Geometry check sheet. Reference: the model listing, model coordinates, mm. A direction names the side the tool comes from. Coordinates: 2 decimals unless noted, no trailing zeros. Write each loop counter-clockwise with the first axis right and the second up, starting at its lowest first coordinate (ties: lowest second). Pieces come first, ordered by that corner, then holes.
Autodesk Fusion 360 part; units mm, degrees
sketch "Sketch1" plane through (0, 0, 0) normal (0, 0, 1) x (1, 0, 0)
  circle A0 centre (0, 0) radius 23
  circle A1 centre (0, 0) radius 14
  circle A2 centre (0, 0) radius 17
  dimension "d1" = 46
  dimension "d2" = 28
  dimension "d3" = 34
extrude "Extrude1" add sketch "Sketch1" along normal blind 3 contours A0 | A2
extrude "Extrude2" add sketch "Sketch1" against normal blind 8 contours A2
1. Sectioned sample at A-A, the plane y = 0. Record the boundary of the cut face in (x, z), and give its area (3 significant figures).
Computed values:
outline: (-23, 0) - (-17, 0) - (-17, -8) - (-14, -8) - (-14, 3) - (-23, 3) - close; (14, -8) - (17, -8) - (17, 0) - (23, 0) - (23, 3) - (14, 3) - close
area: 102 mm2
2. Sectioned sample at B-B, the plane x = 12. Record the boundary of the cut face in (y, z), and give its area (3 significant figures).
Computed values:
outline: (-19.62, 0) - (-12.04, 0) - (-12.04, -8) - (-7.21, -8) - (-7.21, 3) - (-19.62, 3) - close; (7.21, -8) - (12.04, -8) - (12.04, 0) - (19.62, 0) - (19.62, 3) - (7.21, 3) - close
area: 152 mm2
3. Gauge pin test, flat ends, axial feed: pin 1 Ø3 at (x, z) = (16, -0.5) entering from -Y; pin 2 Ø1 at (y, z) = (14, -4) entering from -X; pin 3 Ø5 at (x, y) = (-11, -17) entering from -Z. Record the tip position at first contact, or that the pin passes through.
Computed values:
pin 1: stops at y = -17.78
pin 2: stops at x = -10.33
pin 3: stops at z = 0
4. Access from +Z, -Z, +X, -X, +Y, -Y to the whole of each face (thin tool, end or side, straight path). Record for faces 1 (the cylindrical face through (-2.994, -22.804, 1.479)), 2 (the cylindrical face through (9.139, 14.334, -3.944)).
Computed values:
face 1: +Z, -Z
face 2: -Z
5. Sectioned sample at C-C, the plane y = 15. Record the boundary of the cut face in (x, z), and give its area (3 significant figures).
Computed values:
outline: (-17.44, 0) - (-8, 0) - (-8, -8) - (8, -8) - (8, 0) - (17.44, 0) - (17.44, 3) - (-17.44, 3) - close
area: 233 mm2
6. Thickness scan on line 1 along Y through (x, z) = (0, -3); line 2 along X through (y, z) = (0.5, 0.5); line 3 along X through (y, z) = (-8.5, -7.5). Record the ranges inside material, lowest first.
Computed values:
line 1: y = -17 to -14, 14 to 17
line 2: x = -22.99 to -13.99, 13.99 to 22.99
line 3: x = -14.72 to -11.12, 11.12 to 14.72
